Read the model definition and answer for the solid it produces. Units are mm, in the model's axes. Face numbers are marked on the shaded views. A direction names the side the tool comes from. Give positions to 0.01 mm unless a question says otherwise; leave off trailing zeros. Loops run counter-clockwise (first coordinate to the right, second up) from the corner with the lowest first, then second, coordinate; pieces in that order, holes last. Notation, with made-up numbers: (67, 71) - (101, 71) arc R33 ccw to (101, 109) - close; hole circle Ø4 at (74, 43). An arc over 180 degrees is marked (long way). Write item = value, one per line.
```python
from build123d import *

# Parameters (mm, degrees)
F1_DEPTH = 25


with BuildPart() as f1:
    # F0 (on Right) → F1 (new body)
    with BuildSketch(Plane.YZ):
        with BuildLine():
            Line((-20, -7.5), (20, -7.5))
            Line((20, -7.5), (20, 7.5))
            Line((20, 7.5), (17, 7.5))
            Line((17, 7.5), (17, 2.318182))
            ThreePointArc((17, 2.318182), (9, -3.5), (1, 2.318182))
            Line((1, 2.318182), (1, 7.5))
            Line((1, 7.5), (-1, 7.5))
            Line((-1, 7.5), (-1, 2.318182))
            ThreePointArc((-1, 2.318182), (-9, -3.5), (-17, 2.318182))
            Line((-17, 2.318182), (-17, 7.5))
            Line((-17, 7.5), (-20, 7.5))
            Line((-20, 7.5), (-20, -7.5))
        make_face()
    extrude(amount=F1_DEPTH)


solid = f1.part
```
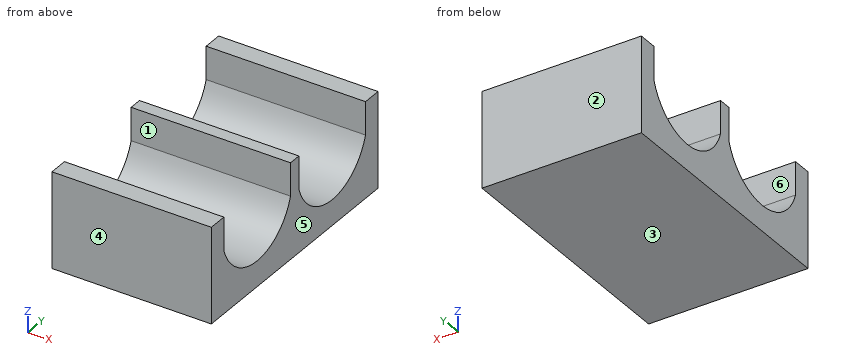
1) A cutting plane is placed at A-A on z = 6. Determine the outline of the cut face in (x, y), then the cut area to 3 significant figures.
Output:
outline = (0, -20) - (25, -20) - (25, -17) - (0, -17) - close; (0, -1) - (25, -1) - (25, 1) - (0, 1) - close; (0, 17) - (25, 17) - (25, 20) - (0, 20) - close
area = 200 mm²
2) A cutting plane is placed at D-D on z = -0.75. Determine the outline of the cut face in (x, y).
Output:
outline = (0, -20) - (25, -20) - (25, -15.22) - (0, -15.22) - close; (0, -2.78) - (25, -2.78) - (25, 2.78) - (0, 2.78) - close; (0, 15.22) - (25, 15.22) - (25, 20) - (0, 20) - close
3) A tool of negligible diameter and unlimited length cuts with its end or side. For the marked faces 5 and 6, from which of +Z, -Z, +X, -X, +Y, -Y can it reach the whole face along a straight path? Write none if from no direction.
Output:
face_5 = +Z, -Z, +X, +Y, -Y
face_6 = +Z, +X, -X
4) A cutting plane is placed at C-C on y = 12.5. Determine the outline of the cut face in (x, z).
Output:
outline = (0, -7.5) - (25, -7.5) - (25, -2.74) - (0, -2.74) - close
5) The mould has two halves that part along Y. Classify the marked faces 1, 2, 3 and 4: pulls with the +Y half, pulls with the -Y half, needs draft (parallel to the pull), parting line crosses it, or undercut.
Output:
face_1 = undercut
face_2 = pulls with the +Y half
face_3 = needs draft
face_4 = pulls with the -Y half
6) Each of these flat-tipped pins is pushed along its axis until it touches: P1, Ø2, axis at x = 17.5, y = 12, coming from the +Z side; P2, Ø4, axis at x = 22, y = 7.5, coming from the +Z side. Where does it stop, or does it pass through?
Output:
P1 = -2.49
P2 = -2.74
7) Find the intervals of material crossed by probe 1 along Y at (x, z) = (16.75, 4.75); probe 2 along Y at (x, z) = (19, -2.25); probe 3 along Z at (x, y) = (17.5, 10.5), in increasing order.
Output:
probe_1 = -20 to -17, -1 to 1, 17 to 20
probe_2 = -20 to -13.41, -4.59 to 4.59, 13.41 to 20
probe_3 = -7.5 to -3.37
8) A cutting plane is placed at B-B on x = 5.75. Determine the outline of the cut face in (y, z).
Output:
outline = (-20, -7.5) - (20, -7.5) - (20, 7.5) - (17, 7.5) - (17, 2.32) arc R8.41 cw to (1, 2.32) - (1, 7.5) - (-1, 7.5) - (-1, 2.32) arc R8.41 cw to (-17, 2.32) - (-17, 7.5) - (-20, 7.5) - close
